```python
from build123d import *

# Parameters (mm, degrees)
BOSS_EXTRUDE1_DEPTH   = 14
CHAMFER1_SIZE         = 0.5
M6X1_0_TAPPED_HOLE1_D = 5


with BuildPart() as part:
    # Sketch1 → Boss-Extrude1 (new body)
    with BuildSketch(Plane.XY):
        with BuildLine():
            Line((-21, 4), (-21, 0))
            Line((-21, 0), (21, 0))
            Line((21, 0), (21, 4))
            ThreePointArc((21, 4), (20.414213562, 5.414213562), (19, 6))
            Line((19, 6), (11, 6))
            ThreePointArc((11, 6), (9.585786438, 6.585786438), (9, 8))
            Line((9, 8), (9, 30.8))
            ThreePointArc((9, 30.8), (8.414213562, 32.214213562), (7, 32.8))
            Line((7, 32.8), (1, 32.8))
            Line((1, 32.8), (1, 23.872983346))
            ThreePointArc((1, 23.872983346), (0, 16), (-1, 23.872983346))
            Line((-1, 23.872983346), (-1, 32.8))
            Line((-1, 32.8), (-7, 32.8))
            ThreePointArc((-7, 32.8), (-8.414213562, 32.214213562), (-9, 30.8))
            Line((-9, 30.8), (-9, 8))
            ThreePointArc((-9, 8), (-9.585786438, 6.585786438), (-11, 6))
            Line((-11, 6), (-19, 6))
            ThreePointArc((-19, 6), (-20.414213562, 5.414213562), (-21, 4))
        make_face()
    extrude(amount=BOSS_EXTRUDE1_DEPTH)

    # Chamfer1
    chamfer1_edges = [part.edges().sort_by_distance(p)[0] for p in [
        (0, 16, 0),
        (0, 16, 14),
    ]]
    chamfer(chamfer1_edges, length=CHAMFER1_SIZE)

    # M6x1.0 Tapped Hole1 (through all)
    with Locations(Plane(origin=(0, 6, 0), x_dir=(1, 0, 0), z_dir=(0, 1, 0))):
        with Locations((-16, -7), (16, -7)):
            Hole(M6X1_0_TAPPED_HOLE1_D / 2)


solid = part.part
```
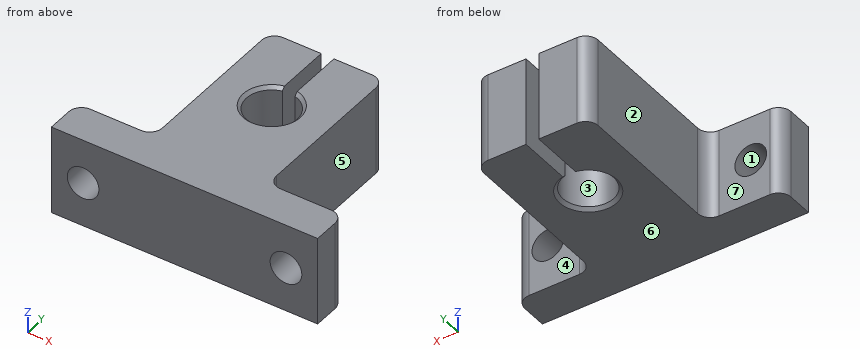
Source: CAD feature listing. Evaluate the final solid. Frame: model axes, mm. Face numbers are marked on the shaded views. A direction names the side the tool comes from. Give positions to 0.01 mm unless a question says otherwise; leave off trailing zeros. Write each loop counter-clockwise with the first axis right and the second up, starting at its lowest first coordinate (ties: lowest second). Pieces come first, ordered by that corner, then holes. Notation, with made-up numbers: (60.5, 64) - (115.5, 64) arc R19 ccw to (115.5, 101) - close; hole circle Ø3 at (88.25, 23.5). An arc over 180 degrees is marked (long way). One line per item, written item: value. Start each with the question number.
Q1. Draft query along X for the marked faces 1, 2, 3 and 4. Return one class per face: +X half, -X half, draft (parallel to the pull), parting line (faces both ways), or undercut.
Q2. Set-up query: the marked faces 5, 6 and 7. Return all of +Z, -Z, +X, -X, +Y, -Y with unobstructed straight access to the full face (end or side cutting, diameter ignored); none if empty.
Q3. First-contact query: pin 1 Ø5 at (y, z) = (22, 9.5) entering from +X; pin 2 Ø3 at (x, z) = (-16, 7) entering from +Y; pin 3 Ø6.5 at (x, z) = (13.5, 6.5) entering from +Y; pin 4 Ø4.5 at (y, z) = (26.5, 10) entering from -X. Flat tips, straight axial feed; report the tip coordinate or a pass-through.
Q4. Section query A-A, the plane y = 29.5. Return the cut outline in (x, z).
Q5. Section query C-C, the plane x = 16. Return the cut outline in (y, z), then the cut area to 3 significant figures.
Q6. Section query D-D, the plane y = 3. Return the cut outline in (x, z), then the cut area to 3 significant figures.
Q7. Material intervals for probe 1 along X at (y, z) = (20, 6); probe 2 along X at (y, z) = (27, 8); probe 3 along Z at (x, y) = (16, 2.7), sorted ascending. Write a range as from..to.
Q8. Section query B-B, the plane z = 8.5. Return the cut outline in (x, y), then the cut area to 3 significant figures.
Answer:
1. face 1: undercut
1. face 2: -X half
1. face 3: undercut
1. face 4: draft
2. face 5: +Z, -Z, +X, +Y
2. face 6: -Z, +X, -X, +Y, -Y
2. face 7: +Z, -Z, -X, +Y
3. pin 1: stops at x = 9
3. pin 2: passes through
3. pin 3: stops at y = 6.15
3. pin 4: stops at x = -9
4. outline: (-9, 0) - (-1, 0) - (-1, 14) - (-9, 14) - close; (1, 0) - (9, 0) - (9, 14) - (1, 14) - close
5. outline: (0, 0) - (6, 0) - (6, 4.5) - (0, 4.5) - close; (0, 9.5) - (6, 9.5) - (6, 14) - (0, 14) - close
5. area: 54.0 mm2
6. outline: (-21, 0) - (21, 0) - (21, 14) - (-21, 14) - close; hole circle Ø5 at (-16, 7); hole circle Ø5 at (16, 7)
6. area: 549 mm2
7. probe 1: x = -9..-4, 4..9
7. probe 2: x = -9..-1, 1..9
7. probe 3: z = 0..4.5, 9.5..14
8. outline: (-21, 0) - (-18, 0) - (-18, 6) - (-19, 6) arc R2 ccw to (-21, 4) - close; (-14, 0) - (14, 0) - (14, 6) - (11, 6) arc R2 cw to (9, 8) - (9, 30.8) arc R2 ccw to (7, 32.8) - (1, 32.8) - (1, 23.87) arc R4 cw (long way) to (-1, 23.87) - (-1, 32.8) - (-7, 32.8) arc R2 ccw to (-9, 30.8) - (-9, 8) arc R2 cw to (-11, 6) - (-14, 6) - close; (18, 0) - (21, 0) - (21, 4) arc R2 ccw to (19, 6) - (18, 6) - close
8. area: 617 mm2
